```python
from build123d import *

# Parameters (mm, degrees)
BASE_DEPTH                      = 418
CHAMFER1_SIZE                   = 3
F_3_2_3_2_CABLE_CARRIER_HOLES_D = 3.2
F_3_2_3_2_DIAMETER_HOLE2_D      = 3.2
F_4_0_4_CABLE_TIE_HOLES_D       = 4


with BuildPart() as part:
    # Sketch1 → Base (new body)
    with BuildSketch(Plane.XY):
        Polygon((0, 0), (20, 0), (20, 1), (1, 1), (1, 20), (0, 20), align=None)
    extrude(amount=BASE_DEPTH)

    # Chamfer1
    chamfer1_edges = [part.edges().sort_by_distance(p)[0] for p in [
        (20, 0.5, 418),
        (0.5, 20, 418),
        (0.5, 20, 0),
        (20, 0.5, 0),
    ]]
    chamfer(chamfer1_edges, length=CHAMFER1_SIZE)

    # Ø3.2 (3.2) Cable Carrier Holes (through all)
    with Locations(Plane(origin=(1, 0, 0), x_dir=(0, 0, -1), z_dir=(1, 0, 0))):
        with Locations((-168.7, 14.85), (-160.9, 7.35)):
            Hole(F_3_2_3_2_CABLE_CARRIER_HOLES_D / 2)

    # Ø3.2 (3.2) Diameter Hole2 (through all)
    with Locations(Plane(origin=(0, 1, 0), x_dir=(1, 0, 0), z_dir=(0, 1, 0))):
        with Locations((7.25, -401.5), (14.75, -407.5), (7.25, -10.5), (14.75, -16.5)):
            Hole(F_3_2_3_2_DIAMETER_HOLE2_D / 2)

    # Ø4.0 (4) Cable Tie Holes (through all)
    with Locations(Plane(origin=(0, 1, 0), x_dir=(1, 0, 0), z_dir=(0, 1, 0))):
        with Locations((11, -25), (11, -135)):
            Hole(F_4_0_4_CABLE_TIE_HOLES_D / 2)


solid = part.part
```
Check sheet for the modelled part. Datum: model origin and axes. Units: mm. A direction names the side the tool comes from. Round coordinates to 2 decimals unless told otherwise and drop trailing zeros. Loops run counter-clockwise (first coordinate to the right, second up) from the corner with the lowest first, then second, coordinate; pieces in that order, holes last. Notation, with made-up numbers: (31, 76.25) -> (86, 76.25) arc R4 ccw to (86, 83.25) -> close; hole circle Ø3 at (76, 1). An arc over 180 degrees is marked (long way). Answer in a Markdown table with one row per item.
Q1. Go/stop test with flat-tipped pins: P1, Ø3, axis at x = 14.75, z = 407.5, coming from the +Y side; P2, Ø4, axis at x = 11, z = 294.5, coming from the +Y side. Record where each tip stops, or that it passes through.
Data:
| item | result |
|---|---|
| P1 | passes through |
| P2 | stops at y = 1 |
Q2. Set-up check for faces 1 (the face through (11, 1, 206)), 2 (the face through (0, 10, 206)): record each of +Z, -Z, +X, -X, +Y, -Y from which the full face is reachable in a straight line by a thin tool's end or side.
Data:
| item | result |
|---|---|
| face 1 | +Z, -Z, +X, +Y |
| face 2 | +Z, -Z, -X, +Y, -Y |
Q3. Thickness scan on L1, parallel to Z at x = 11, y = 0.8; L2, parallel to Z at x = 7.25, y = 0.8; L3, parallel to X at y = 0.2, z = 407.5. Record the ranges inside material, lowest first.
Data:
| item | result |
|---|---|
| L1 | z = 0 to 23, 27 to 133, 137 to 418 |
| L2 | z = 0 to 8.9, 12.1 to 399.9, 403.1 to 418 |
| L3 | x = 0 to 13.15, 16.35 to 20 |
Q4. Sectioned sample at A-A on z = 232. Enter the section's corners in (x, y), then the cut area to 3 significant figures.
Data:
| item | result |
|---|---|
| outline | (0, 0) -> (20, 0) -> (20, 1) -> (1, 1) -> (1, 20) -> (0, 20) -> close |
| area | 39.0 mm^2 |
